from build123d import *

# Parameters (mm, degrees)
F0_R     = 3.2
F0_W     = 12.2
F0_H     = 10.2
F1_DEPTH = 7.8
F2_START = 0.8
F0_R_2   = 2.4
F2_DEPTH = 6.2
F0_R_3   = 1
F0_R_4   = 2
F3_DEPTH = 0.8


with BuildPart() as f1:
    # F0 (on Top) → F1 (new body)
    with BuildSketch(Plane.XY):
        with BuildLine():
            Line((12, 7.7), (-12, 7.7))
            ThreePointArc((-12, 7.7), (-14.6162950904, 6.6162950904), (-15.7, 4))
            Line((-15.7, 4), (-15.7, -4))
            ThreePointArc((-15.7, -4), (-14.6162950904, -6.6162950904), (-12, -7.7))
            Line((-12, -7.7), (12, -7.7))
            ThreePointArc((12, -7.7), (14.6162950904, -6.6162950904), (15.7, -4))
            Line((15.7, -4), (15.7, 4))
            ThreePointArc((15.7, 4), (14.6162950904, 6.6162950904), (12, 7.7))
        make_face()
        with Locations((-12, -4)):
            Circle(F0_R, mode=Mode.SUBTRACT)
        with Locations((12, -4)):
            Circle(F0_R, mode=Mode.SUBTRACT)
        with Locations((-12, 4)):
            Circle(F0_R, mode=Mode.SUBTRACT)
        Rectangle(F0_W, F0_H, mode=Mode.SUBTRACT)
        with Locations((12, 4)):
            Circle(F0_R, mode=Mode.SUBTRACT)
    extrude(amount=F1_DEPTH)

    # F0 (on Top) → F2 (join)
    with BuildSketch(Plane.XY.offset(F2_START)):
        with Locations((-12, -4)):
            Circle(F0_R)
        with Locations((-12, -4)):
            Circle(F0_R_2, mode=Mode.SUBTRACT)
        with Locations((12, -4)):
            Circle(F0_R)
        with Locations((12, -4)):
            Circle(F0_R_2, mode=Mode.SUBTRACT)
        with Locations((-12, 4)):
            Circle(F0_R)
        with Locations((-12, 4)):
            Circle(F0_R_2, mode=Mode.SUBTRACT)
        with Locations((12, 4)):
            Circle(F0_R)
        with Locations((12, 4)):
            Circle(F0_R_2, mode=Mode.SUBTRACT)
    extrude(amount=F2_DEPTH)

    # F0 (on Top) → F3 (join)
    with BuildSketch(Plane.XY):
        Rectangle(F0_W, F0_H)
        with Locations((-4.5, 0)):
            Circle(F0_R_3, mode=Mode.SUBTRACT)
        Circle(F0_R_4, mode=Mode.SUBTRACT)
        with Locations((4.5, 0)):
            Circle(F0_R_3, mode=Mode.SUBTRACT)
    extrude(amount=F3_DEPTH)


solid = f1.part
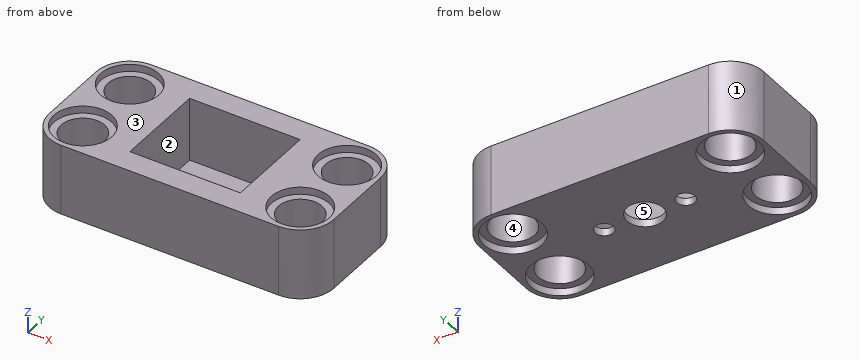
Design review of the part built by this model. Coordinates are the model's own, in mm. Face numbers are marked on the shaded views. A direction names the side the tool comes from. Coordinates: 2 decimals unless noted, no trailing zeros. Loops run counter-clockwise (first coordinate to the right, second up) from the corner with the lowest first, then second, coordinate; pieces in that order, holes last.
Item 1: Draft analysis for pull direction X (two halves, no side actions). For the marked faces 1, 2 and 3, state which applies: pulls with the +X half, pulls with the -X half, needs draft (parallel to the pull), parting line crosses it, or undercut.
Completed:
face 1: pulls with the -X half
face 2: undercut
face 3: needs draft
Item 2: Add section C-C (z = 4.75). Write out the cut boundary in (x, y), and give its area (3 significant figures).
Completed:
outline: (-15.7, -4) arc R3.7 ccw to (-12, -7.7) - (12, -7.7) arc R3.7 ccw to (15.7, -4) - (15.7, 4) arc R3.7 ccw to (12, 7.7) - (-12, 7.7) arc R3.7 ccw to (-15.7, 4) - close; hole circle Ø4.8 at (-12, -4); hole circle Ø4.8 at (-12, 4); hole (-6.1, -5.1) - (6.1, -5.1) - (6.1, 5.1) - (-6.1, 5.1) - close; hole circle Ø4.8 at (12, -4); hole circle Ø4.8 at (12, 4)
area: 275 mm2
Item 3: Add section A-A (y = 0). Write out the cut boundary in (x, z).
Completed:
outline: (-15.7, 0) - (-5.5, 0) - (-5.5, 0.8) - (-6.1, 0.8) - (-6.1, 7.8) - (-15.7, 7.8) - close; (-3.5, 0) - (-2, 0) - (-2, 0.8) - (-3.5, 0.8) - close; (2, 0) - (3.5, 0) - (3.5, 0.8) - (2, 0.8) - close; (5.5, 0) - (15.7, 0) - (15.7, 7.8) - (6.1, 7.8) - (6.1, 0.8) - (5.5, 0.8) - close
Item 4: For the marked faces 4 and 5, list the 3-axis set-ups (+Z, -Z, +X, -X, +Y, -Y) from which the entire face can be reached by the end or side of a thin tool; tool diameter is ignored.
Completed:
face 4: +Z, -Z
face 5: +Z
Item 5: Add section B-B (x = -4.5). Write out the cut boundary in (y, z), and give its area (3 significant figures).
Completed:
outline: (-7.7, 0) - (-1, 0) - (-1, 0.8) - (-5.1, 0.8) - (-5.1, 7.8) - (-7.7, 7.8) - close; (1, 0) - (7.7, 0) - (7.7, 7.8) - (5.1, 7.8) - (5.1, 0.8) - (1, 0.8) - close
area: 47.1 mm2
Item 6: Add section D-D (x = -13). Write out the cut boundary in (y, z).
Completed:
outline: (-7.56, 0) - (-7.04, 0) - (-7.04, 0.8) - (-6.18, 0.8) - (-6.18, 7) - (-7.04, 7) - (-7.04, 7.8) - (-7.56, 7.8) - close; (-1.82, 0.8) - (-0.96, 0.8) - (-0.96, 0) - (0.96, 0) - (0.96, 0.8) - (1.82, 0.8) - (1.82, 7) - (0.96, 7) - (0.96, 7.8) - (-0.96, 7.8) - (-0.96, 7) - (-1.82, 7) - close; (6.18, 0.8) - (7.04, 0.8) - (7.04, 0) - (7.56, 0) - (7.56, 7.8) - (7.04, 7.8) - (7.04, 7) - (6.18, 7) - close
Item 7: Wall thickness on L1, parallel to Y at x = -6, z = 6.5; L2, parallel to Y at x = 12, z = 0.3; L3, parallel to X at y = 4.5, z = 5.5: over which ranges is each line inside the solid? List them lowest first.
Completed:
L1: y = -7.7 to -5.1, 5.1 to 7.7
L2: y = -7.7 to -7.2, -0.8 to 0.8, 7.2 to 7.7
L3: x = -15.67 to -14.35, -9.65 to -6.1, 6.1 to 9.65, 14.35 to 15.67
Item 8: Clearance check with flat-ended pins moving along their axes: pin 1 (1.6 mm diameter, centred on x = 4.5, y = 0, fed in from +Z); pin 2 (5 mm diameter, centred on x = 13.5, y = -3.5, fed in from +Z); pin 3 (3 mm diameter, centred on x = 13, y = 4, fed in from -Z); pin 4 (2 mm diameter, centred on y = 5.5, z = 2, fed in from -X). State where each tip first meets the part, or that it passes through.
Completed:
pin 1: passes through
pin 2: stops at z = 7.8
pin 3: stops at z = 0.8
pin 4: stops at x = -15.67
